```python
from build123d import *

# Parameters (mm, degrees)
SKETCH1_W           = 50
SKETCH1_H           = 35
BOSS_EXTRUDE1_DEPTH = 45
SKETCH3_W           = 45
SKETCH3_H           = 11.666666667
CUT_EXTRUDE2_DEPTH  = 76.828754441
SHELL1_T            = -2.5
SKETCH2_R           = 3.5
SKETCH2_R_2         = 2.35
CUT_EXTRUDE1_DEPTH  = 4
SKETCH4_W           = 46.6
SKETCH4_H           = 41.6
SKETCH4_W_2         = 45
SKETCH4_H_2         = 40
BOSS_EXTRUDE2_DEPTH = 2.5
FILLET1_R           = 3
FILLET2_R           = 1
CHAMFER1_SIZE       = 1.5
FILLET3_R           = 1


with BuildPart() as part:
    # Sketch1 → Boss-Extrude1 (new body)
    with BuildSketch(Plane.XY):
        with Locations((25, 17.5)):
            Rectangle(SKETCH1_W, SKETCH1_H)
    extrude(amount=BOSS_EXTRUDE1_DEPTH)

    # Sketch3 → Cut-Extrude2 (cut, through all)
    with BuildSketch(Plane(origin=(50, 0, 0), x_dir=(0, 0, -1), z_dir=(1, 0, 0))):
        with Locations((-22.5, 29.166666666)):
            Rectangle(SKETCH3_W, SKETCH3_H)
    extrude(amount=-CUT_EXTRUDE2_DEPTH, mode=Mode.SUBTRACT)

    # Shell1
    shell1_openings = [part.faces().sort_by_distance(p)[0] for p in [
        (25, 23.333333333, 22.5),
    ]]
    offset(amount=SHELL1_T, openings=shell1_openings, kind=Kind.INTERSECTION)

    # Sketch2 → Cut-Extrude1 (cut)
    with BuildSketch(Plane(origin=(50, 0, 0), x_dir=(0, 0, -1), z_dir=(1, 0, 0))):
        with Locations((-32.5, 11.666666667)):
            Circle(SKETCH2_R)
        with Locations((-12.5, 11.666666667)):
            Circle(SKETCH2_R_2)
    extrude(amount=-CUT_EXTRUDE1_DEPTH, mode=Mode.SUBTRACT)

    # Sketch4 → Boss-Extrude2 (add)
    with BuildSketch(Plane(origin=(0, 23.333333333, 0), x_dir=(1, 0, 0), z_dir=(0, 1, 0))):
        with Locations((25, -22.5)):
            Rectangle(SKETCH4_W, SKETCH4_H)
        with Locations((25, -22.5)):
            Rectangle(SKETCH4_W_2, SKETCH4_H_2, mode=Mode.SUBTRACT)
    extrude(amount=BOSS_EXTRUDE2_DEPTH)

    # Fillet1
    fillet1_edges = [part.edges().sort_by_distance(p)[0] for p in [
        (50, 11.666666667, 45),
        (0, 11.666666667, 0),
        (0, 11.666666667, 45),
        (50, 11.666666667, 0),
    ]]
    fillet(fillet1_edges, radius=FILLET1_R)

    # Fillet2
    fillet2_edges = [part.edges().sort_by_distance(p)[0] for p in [
        (1.7, 24.583333333, 1.7),
        (1.7, 24.583333333, 43.3),
        (48.3, 24.583333333, 43.3),
        (48.3, 24.583333333, 1.7),
    ]]
    fillet(fillet2_edges, radius=FILLET2_R)

    # Chamfer1
    chamfer1_edges = [part.edges().sort_by_distance(p)[0] for p in [
        (49.121320344, 0, 0.878679656),
        (0.878679656, 0, 0.878679656),
        (0, 0, 22.5),
        (25, 0, 0),
        (50, 0, 22.5),
        (25, 0, 45),
        (0.878679656, 0, 44.121320344),
        (49.121320344, 0, 44.121320344),
    ]]
    chamfer(chamfer1_edges, length=CHAMFER1_SIZE)

    # Fillet3
    fillet3_edges = [part.edges().sort_by_distance(p)[0] for p in [
        (47.5, 11.666666667, 36),
        (47.5, 11.666666667, 14.85),
    ]]
    fillet(fillet3_edges, radius=FILLET3_R)


solid = part.part
```
CAD build for the part. Positions are in the model's coordinates, mm. A direction names the side the tool comes from. Round coordinates to 2 decimals unless told otherwise and drop trailing zeros. Write each loop counter-clockwise with the first axis right and the second up, starting at its lowest first coordinate (ties: lowest second). Pieces come first, ordered by that corner, then holes. Notation, with made-up numbers: (23.5, -28) - (55.5, -28) arc R14 cw to (55.5, -18) - close; hole circle Ø2 at (67, -13.5). An arc over 180 degrees is marked (long way). Write item = value, one per line. Start each with the question number.
Q1. Mould opens along Z. For faces 4 (the flat face through (25, 14, 2.5)), 5 (the flat face through (25, 0, 22)), 6 (the flat face through (25, 2.5, 22)), 7 (the flat face through (25, 13, 0)) say: pulls with the +Z half, pulls with the -Z half, needs draft (parallel to the pull), parting line crosses it, or undercut.
Q2. Band-saw the part on A-A (z = 32.5). Give the cut face in (x, y).
Q3. Band-saw the part on B-B (z = 6.5). Give the cut face in (x, y).
Q4. Band-saw the part on D-D (x = 4). Give the cut face in (y, z), then the cut area to 3 significant figures.
Q5. Probe L1, parallel to X at y = 17.25, z = 26.5; L2, parallel to X at y = 24.5, z = 39; L3, parallel to Z at x = 41, y = 10. List the from-to ranges inside material, lowest first. Write a range as from..to.
Q6. Drop flat-ended pins along their axis: pin 1 (3 mm diameter, centred on x = 22.5, y = 25, fed in from -Z); pin 2 (13.5 mm diameter, centred on x = 33.5, z = 16, fed in from +Y); pin 3 (7 mm diameter, centred on y = 11, z = 30, fed in from +X); pin 4 (2 mm diameter, centred on x = 18.5, y = 25, fed in from +Z). Give the stop position or say it passes through.
Q7. Which spindle directions (+Z, -Z, +X, -X, +Y, -Y) get a long thin tool onto all of the face, cutting with end or side? Do faces 1 (the flat face through (25, 25, 1.7)), 2 (the flat face through (47.5, 14, 23)), 3 (the flat face through (48.3, 25, 23)). Say none if no direction does.
Q8. Band-saw the part on C-C (y = 3.5). Give the cut face in (x, z).
Answers below:
q1.face_4 = undercut
q1.face_5 = needs draft
q1.face_6 = undercut
q1.face_7 = pulls with the -Z half
q2.outline = (0, 1.5) - (1.5, 0) - (48.5, 0) - (50, 1.5) - (50, 8.17) - (48.5, 8.17) arc R1 ccw to (47.5, 7.17) - (47.5, 2.5) - (2.5, 2.5) - (2.5, 25.83) - (1.7, 25.83) - (1.7, 23.33) - (0, 23.33) - close; (47.5, 16.17) arc R1 ccw to (48.5, 15.17) - (50, 15.17) - (50, 23.33) - (48.3, 23.33) - (48.3, 25.83) - (47.5, 25.83) - close
q3.outline = (0, 1.5) - (1.5, 0) - (48.5, 0) - (50, 1.5) - (50, 23.33) - (48.3, 23.33) - (48.3, 25.83) - (47.5, 25.83) - (47.5, 2.5) - (2.5, 2.5) - (2.5, 25.83) - (1.7, 25.83) - (1.7, 23.33) - (0, 23.33) - close
q4.outline = (0, 1.5) - (1.5, 0) - (23.33, 0) - (23.33, 1.7) - (25.83, 1.7) - (25.83, 2.5) - (2.5, 2.5) - (2.5, 42.5) - (25.83, 42.5) - (25.83, 43.3) - (23.33, 43.3) - (23.33, 45) - (1.5, 45) - (0, 43.5) - close
q4.area = 218 mm2
q5.L1 = 0..2.5, 47.5..50
q5.L2 = 1.7..2.5, 47.5..48.3
q5.L3 = 0..2.5, 42.5..45
q6.pin_1 = 1.7
q6.pin_2 = 2.5
q6.pin_3 = 50
q6.pin_4 = 43.3
q7.face_1 = -Z, +X, -X, +Y
q7.face_2 = +Y
q7.face_3 = +Z, -Z, +X, +Y
q8.outline = (0, 3) arc R3 ccw to (3, 0) - (47, 0) arc R3 ccw to (50, 3) - (50, 42) arc R3 ccw to (47, 45) - (3, 45) arc R3 ccw to (0, 42) - close; hole (2.5, 2.5) - (47.5, 2.5) - (47.5, 42.5) - (2.5, 42.5) - close
